Here's how the part is built. I have some questions about the finished solid (model axes, mm). Face numbers are marked on the shaded views. A direction names the side the tool comes from. Round coordinates to 2 decimals unless told otherwise and drop trailing zeros. Loops run counter-clockwise (first coordinate to the right, second up) from the corner with the lowest first, then second, coordinate; pieces in that order, holes last. Notation, with made-up numbers: (6.25, 74.25) - (42.25, 74.25) arc R22 ccw to (42.25, 98.25) - close; hole circle Ø9 at (19, 44.5). An arc over 180 degrees is marked (long way). Return JSON: item names as keys, results as strings. Group by question number.
```python
from build123d import *

# Parameters (mm, degrees)
SKETCH1_W           = 17.4
SKETCH1_H           = 17.4
BOSS_EXTRUDE1_DEPTH = 6.5
FILLET1_R           = 3.5
CUT_EXTRUDE1_DEPTH  = 5.5
SKETCH3_R           = 4
SKETCH3_R_2         = 2.75
BOSS_EXTRUDE2_DEPTH = 5.5
SKETCH4_R           = 2.75
CUT_EXTRUDE2_DEPTH  = 0.4


with BuildPart() as part:
    # Sketch1 → Boss-Extrude1 (new body)
    with BuildSketch(Plane(origin=(0, 0, 0), x_dir=(1, 0, 0), z_dir=(0, 1, 0))):
        with Locations((-8.7, -8.7)):
            Rectangle(SKETCH1_W, SKETCH1_H)
    extrude(amount=BOSS_EXTRUDE1_DEPTH)

    # Fillet1
    fillet1_edges = [part.edges().sort_by_distance(p)[0] for p in [
        (0, 3.25, 17.4),
        (-17.4, 3.25, 17.4),
        (-17.4, 3.25, 0),
        (0, 3.25, 0),
    ]]
    fillet(fillet1_edges, radius=FILLET1_R)

    # Sketch2 → Cut-Extrude1 (cut)
    with BuildSketch(Plane(origin=(0, 6.5, 0), x_dir=(1, 0, 0), z_dir=(0, 1, 0))):
        with BuildLine():
            Line((-13.9, -15.9), (-3.5, -15.9))
            ThreePointArc((-3.5, -15.9), (-2.085786438, -15.314213562), (-1.5, -13.9))
            Line((-1.5, -13.9), (-1.5, -3.5))
            ThreePointArc((-1.5, -3.5), (-2.085786438, -2.085786438), (-3.5, -1.5))
            Line((-3.5, -1.5), (-13.9, -1.5))
            ThreePointArc((-13.9, -1.5), (-15.314213562, -2.085786438), (-15.9, -3.5))
            Line((-15.9, -3.5), (-15.9, -13.9))
            ThreePointArc((-15.9, -13.9), (-15.314213562, -15.314213562), (-13.9, -15.9))
        make_face()
    extrude(amount=-CUT_EXTRUDE1_DEPTH, mode=Mode.SUBTRACT)

    # Sketch3 → Boss-Extrude2 (add)
    with BuildSketch(Plane(origin=(0, 1, 0), x_dir=(1, 0, 0), z_dir=(0, 1, 0))):
        with Locations((-8.7, -8.7)):
            Circle(SKETCH3_R)
        with Locations((-8.7, -8.7)):
            Circle(SKETCH3_R_2, mode=Mode.SUBTRACT)
    extrude(amount=BOSS_EXTRUDE2_DEPTH)

    # Sketch4 → Cut-Extrude2 (cut)
    with BuildSketch(Plane(origin=(0, 1, 0), x_dir=(1, 0, 0), z_dir=(0, 1, 0))):
        with Locations((-8.7, -8.7)):
            Circle(SKETCH4_R)
    extrude(amount=-CUT_EXTRUDE2_DEPTH, mode=Mode.SUBTRACT)


solid = part.part
```
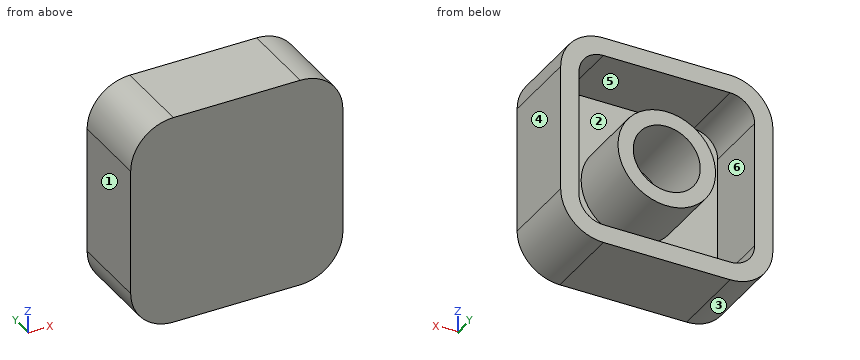
Q1. Imagine slicing it at D-D, the plane z = 8.7. List the corners of the cut face in (x, y) for me.
Q2. Imagine slicing it at C-C, the plane x = -8.7. List the corners of the cut face in (y, z) for me.
Q3. For the marked faces 1 and 2, which set-ups out of +Z, -Z, +X, -X, +Y, -Y let a thin tool reach every point of the face, with its end or its side?
Q4. Will these pins go through, and if not, where does the flat tip stop? pin 1 Ø7 at (x, z) = (-7, 8) entering from +Y; pin 2 Ø1 at (x, y) = (-2, 1) entering from -Z; pin 3 Ø1.6 at (x, z) = (-9, 8.5) entering from +Y.
Q5. If we mould it in two halves opening along Z, with no side actions, what happens to the marked faces 3, 4, 5 and 6? For each: +Z half, -Z half, draft (parallel to the pull), parting line (faces both ways), or undercut.
Q6. Please list where these lines run through material, in increasing order: line 1 (Z direction, x = -8.7, y = 2.55); line 2 (X direction, y = 4.6, z = 8.7); line 3 (X direction, y = 6.25, z = 12.25).
Q7. Imagine slicing it at A-A, the plane y = 4.25. List the corners of the cut face in (x, z) for me, and give its area (3 significant figures).
Q8. Imagine slicing it at B-B, the plane z = 3.75. List the corners of the cut face in (x, y) for me.
Output values:
{
 "1": {"outline": "(-17.4, 0) - (0, 0) - (0, 6.5) - (-1.5, 6.5) - (-1.5, 1) - (-4.7, 1) - (-4.7, 6.5) - (-5.95, 6.5) - (-5.95, 0.6) - (-11.45, 0.6) - (-11.45, 6.5) - (-12.7, 6.5) - (-12.7, 1) - (-15.9, 1) - (-15.9, 6.5) - (-17.4, 6.5) - close"},
 "2": {"outline": "(0, 0) - (6.5, 0) - (6.5, 1.5) - (1, 1.5) - (1, 4.7) - (6.5, 4.7) - (6.5, 5.95) - (0.6, 5.95) - (0.6, 11.45) - (6.5, 11.45) - (6.5, 12.7) - (1, 12.7) - (1, 15.9) - (6.5, 15.9) - (6.5, 17.4) - (0, 17.4) - close"},
 "3": {"face 1": "+Z, -Z, -X, +Y, -Y", "face 2": "+Y"},
 "4": {"pin 1": "stops at y = 6.5", "pin 2": "stops at z = 0.15", "pin 3": "stops at y = 0.6"},
 "5": {"face 3": "-Z half", "face 4": "draft", "face 5": "undercut", "face 6": "undercut"},
 "6": {"line 1": "z = 0 to 1.5, 4.7 to 5.95, 11.45 to 12.7, 15.9 to 17.4", "line 2": "x = -17.4 to -15.9, -12.7 to -11.45, -5.95 to -4.7, -1.5 to 0", "line 3": "x = -17.4 to -15.9, -10.54 to -6.86, -1.5 to 0"},
 "7": {"outline": "(-17.4, 3.5) arc R3.5 ccw to (-13.9, 0) - (-3.5, 0) arc R3.5 ccw to (0, 3.5) - (0, 13.9) arc R3.5 ccw to (-3.5, 17.4) - (-13.9, 17.4) arc R3.5 ccw to (-17.4, 13.9) - close; circle Ø8 at (-8.7, 8.7); hole (-15.9, 3.5) arc R2 ccw to (-13.9, 1.5) - (-3.5, 1.5) arc R2 ccw to (-1.5, 3.5) - (-1.5, 13.9) arc R2 ccw to (-3.5, 15.9) - (-13.9, 15.9) arc R2 ccw to (-15.9, 13.9) - close; hole circle Ø5.5 at (-8.7, 8.7)", "area": "115 mm^2"},
 "8": {"outline": "(-17.4, 0) - (0, 0) - (0, 6.5) - (-1.5, 6.5) - (-1.5, 1) - (-15.9, 1) - (-15.9, 6.5) - (-17.4, 6.5) - close"}
}
